Build history of the part. All positions in model axes, mm. A direction names the side the tool comes from. Give positions to 0.01 mm unless a question says otherwise; leave off trailing zeros. Order: outer loops, then holes, each group sorted by start corner. A loop starts at its lowest first (then second) coordinate and runs counter-clockwise, first axis right, second up. Notation, with made-up numbers: (46, -22.75) -> (95, -22.75) arc R10 ccw to (95, -8.75) -> close; hole circle Ø3 at (10, 86.5). An arc over 180 degrees is marked (long way). One line per question, with ' | ' between items. Start each with the question number.
(1) Pull direction X, two halves, no side cores. Call faces 6 (the face through (-4.36, 8, -3.69)), 7 (the face through (-5.74, 8, -3.3)), 8 (the face through (0, 17.5, 1.703)), 9 (the face through (3.85, 8, 4.13)): +X half, -X half, draft (parallel to the pull), parting line (faces both ways), or undercut.
(2) Cut at B-B (z = 0). Give the cut face in (x, y), then the cut area to 3 significant figures.
(3) Cut at C-C (x = -5). Give the cut face in (y, z), then the cut area to 3 significant figures.
(4) Cut at D-D (y = 14). Give the cut face in (x, z).
(5) Drill centre lines: L1, parallel to Y at x = 1, z = -1.75; L2, parallel to Y at x = 4, z = 3.75; L3, parallel to X at y = 11.25, z = 4. Where is each one in solid material? Low to high. Write a range as from..to.
(6) Which spindle directions (+Z, -Z, +X, -X, +Y, -Y) get a long thin tool onto all of the face, cutting with end or side? Do faces 1 (the face through (-1.454, 17.511, -0.887)), 2 (the face through (0, 18.018, 0)), 3 (the face through (1.496, 17.511, -0.816)), 4 (the face through (5, 9.018, 3)), 5 (the face through (1.4, 7.018, 3.1)). Say none if no direction does.
(7) Cut at A-A (y = 7.5). Give the cut face in (x, z).
(8) Pin check, flat tips, straight feed: pin 1 Ø2 at (x, z) = (-5, -3) entering from +Y; pin 2 Ø4 at (x, y) = (-3, 15) entering from +Z; pin 3 Ø2 at (x, y) = (-2, 4) entering from -Z. Stop position of each tip, or through.
from build123d import *

# Parameters (mm, degrees)
SKETCH1_R           = 3.25
BOSS_EXTRUDE1_DEPTH = 7.018
SKETCH6_R           = 4.7
BOSS_EXTRUDE2_DEPTH = 10
BOSS_EXTRUDE5_DEPTH = 1
FILLET1_R           = 0.75
BOSS_EXTRUDE6_DEPTH = 2


with BuildPart() as part:
    # Sketch1 → Boss-Extrude1 (new body)
    with BuildSketch(Plane(origin=(0, 0, 0), x_dir=(1, 0, 0), z_dir=(0, 1, 0))):
        Circle(SKETCH1_R)
    extrude(amount=BOSS_EXTRUDE1_DEPTH)

    # Sketch6 → Boss-Extrude2 (add)
    with BuildSketch(Plane(origin=(0, 7.018, 0), x_dir=(1, 0, 0), z_dir=(0, 1, 0))):
        Circle(SKETCH6_R)
    extrude(amount=BOSS_EXTRUDE2_DEPTH)

    # Sketch7 → Boss-Extrude5 (add)
    with BuildSketch(Plane(origin=(0, 17.018, 0), x_dir=(1, 0, 0), z_dir=(0, 1, 0))):
        Polygon((2.95, -1.703183294), (0, 3.406366588), (-2.95, -1.703183294), align=None)
    extrude(amount=BOSS_EXTRUDE5_DEPTH)

    # Fillet1
    fillet1_edges = [part.edges().sort_by_distance(p)[0] for p in [
        (-4.7, 17.018, 0),
    ]]
    fillet(fillet1_edges, radius=FILLET1_R)

    # Sketch8 → Boss-Extrude6 (add)
    with BuildSketch(Plane.XZ.offset(-7.018)):
        with BuildLine():
            Line((-4.482079516, -1.414554068), (-6.241843137, -2.430554068))
            Line((-6.241843137, -2.430554068), (-5.225843137, -4.190317689))
            Line((-5.225843137, -4.190317689), (-3.466079516, -3.174317689))
            ThreePointArc((-3.466079516, -3.174317689), (-4.070319398, -2.35), (-4.482079516, -1.414554068))
        make_face()
        with BuildLine():
            Line((2.985424986, 3.630046508), (4.745188607, 4.646046508))
            Line((4.745188607, 4.646046508), (6.396188607, 1.786430625))
            Line((6.396188607, 1.786430625), (4.636424986, 0.770430625))
            ThreePointArc((4.636424986, 0.770430625), (4.070319398, 2.35), (2.985424986, 3.630046508))
        make_face()
    extrude(amount=-BOSS_EXTRUDE6_DEPTH)


solid = part.part
Result set:
1) face 6: undercut | face 7: -X half | face 8: draft | face 9: undercut
2) outline: (-4.7, 7.02) -> (-3.25, 7.02) -> (-3.25, 0) -> (3.25, 0) -> (3.25, 7.02) -> (4.7, 7.02) -> (4.7, 16.27) arc R0.75 ccw to (3.95, 17.02) -> (1.97, 17.02) -> (1.97, 18.02) -> (-1.97, 18.02) -> (-1.97, 17.02) -> (-3.95, 17.02) arc R0.75 ccw to (-4.7, 16.27) -> close | area: 143 mm2
3) outline: (7.02, -4.06) -> (9.02, -4.06) -> (9.02, -1.71) -> (7.02, -1.71) -> close | area: 4.69 mm2
4) outline: circle Ø9.4 at (0, 0)
5) L1: y = 0..17.02 | L2: y = 7.02..9.02 | L3: x = -2.47..2.47
6) face 1: -Z, -X, +Y | face 2: +Z, -Z, +X, -X, +Y | face 3: -Z, +X, +Y | face 4: +Z, +X, +Y | face 5: -Y
7) outline: (-6.24, -2.43) -> (-5.23, -4.19) -> (-3.47, -3.17) arc R4.7 ccw to (4.64, 0.77) -> (6.4, 1.79) -> (4.75, 4.65) -> (2.99, 3.63) arc R4.7 ccw to (-4.48, -1.41) -> close
8) pin 1: stops at y = 9.02 | pin 2: stops at z = 4.59 | pin 3: stops at z = -3.09
